Part model, mm, in its own coordinate system. Face numbers are marked on the shaded views. A direction names the side the tool comes from. Round coordinates to 2 decimals unless told otherwise and drop trailing zeros. Write each loop counter-clockwise with the first axis right and the second up, starting at its lowest first coordinate (ties: lowest second). Pieces come first, ordered by that corner, then holes. Notation, with made-up numbers: M 87.25,77.5 L 145.25,77.5 A18 cw 145.25,95.5 Z; hole C 15.25,47 d4. An arc over 180 degrees is marked long. Use a Markdown table: item, result. Add a question column.
1) Slice it at C-C on y = 43.75. Write the cut outline in (x, z), plus the area to 3 significant figures.
2) Two-plate mould, pull along X, no slides. Class the marked faces 4, 5 and 6: released by +X, released by -X, zero draft, split by the parting line, or undercut.
3) Drop flat-ended pins along their axis: P1, Ø4, axis at x = -39.55, y = 45.99, coming from the +Z side; P2, Ø4, axis at x = -41, y = 45.5, coming from the +Z side; P3, Ø2, axis at x = -64.48, y = 45.99, coming from the +Z side; P4, Ø1, axis at x = -54.5, z = 2.5, coming from the +Y side. Give the stop position or say it passes through.
4) Slice it at B-B on x = -48. Write the cut outline in (y, z).
5) Which spindle directions (+Z, -Z, +X, -X, +Y, -Y) get a long thin tool onto all of the face, cutting with end or side? Do the marked faces 1, 2 and 3. Say none if no direction does.
6) Slice it at A-A on y = 45. Write the cut outline in (x, z).
7) Wall check: probe 1 along X at (y, z) = (44.5, 1.45); probe 2 along X at (y, z) = (44, 1.45); probe 3 along Y at (x, z) = (-39, 1.1). Give the ranges that are in metal, low to high.
8) Slice it at D-D on z = 1.5. Write the cut outline in (x, y), plus the area to 3 significant figures.
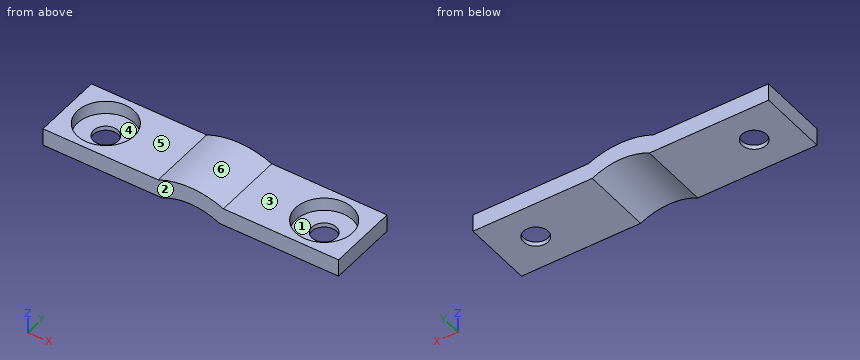
```python
from build123d import *

# Parameters (mm, degrees)
SALIENTE_EXTRUIR3_DEPTH = 4
CROQUIS4_W              = 2
CROQUIS4_H              = 8
SALIENTE_EXTRUIR5_DEPTH = 13.154785
CROQUIS5_R              = 3.25
CORTAR_EXTRUIR1_DEPTH   = 1.5
CORTAR_EXTRUIR2_REACH   = 2.5
CROQUIS6_R              = 1.4


with BuildPart() as part:
    # Croquis3 → Saliente-Extruir3 (new body, symmetric)
    with BuildSketch(Plane(origin=(0, 45.994416346, 0), x_dir=(1, 0, 0), z_dir=(0, 1, 0))):
        with BuildLine():
            ThreePointArc((-58.564503824, 0), (-52.019276555, -2.8), (-45.474049286, 0))
            Line((-45.474049286, 0), (-48.757375269, 0))
            ThreePointArc((-48.757375269, 0), (-52.019276555, -0.8), (-55.281177841, 0))
            Line((-55.281177841, 0), (-58.564503824, 0))
        make_face()
    extrude(amount=SALIENTE_EXTRUIR3_DEPTH, both=True)

    # Croquis4 → Saliente-Extruir5 (add)
    with BuildSketch(Plane(origin=(-68.894276555, 0, 0), x_dir=(0, 0, -1), z_dir=(1, 0, 0))):
        with Locations((-1, 45.994416346)):
            Rectangle(CROQUIS4_W, CROQUIS4_H)
    saliente_extruir5 = extrude(amount=SALIENTE_EXTRUIR5_DEPTH)

    # Simetría1: Saliente-Extruir5 across plane
    add(saliente_extruir5.mirror(Plane(origin=(-52.019276555, 0, 0), x_dir=(0, 0, 1), z_dir=(1, 0, 0))))

    # Croquis5 → Cortar-Extruir1 (cut)
    with BuildSketch(Plane.XY.offset(2)):
        with Locations((-39.554276555, 45.994416346)):
            Circle(CROQUIS5_R)
        with Locations((-64.484276555, 45.994416346)):
            Circle(CROQUIS5_R)
    extrude(amount=-CORTAR_EXTRUIR1_DEPTH, mode=Mode.SUBTRACT)

    # Croquis6 → Cortar-Extruir2 (cut, up to next)
    with BuildSketch(Plane.XY.offset(0.5), mode=Mode.PRIVATE) as cortar_extruir2_sk1:
        with Locations((-39.554276555, 45.994416346)):
            Circle(CROQUIS6_R)
    cortar_extruir2_tool1 = extrude(cortar_extruir2_sk1.sketch, amount=-CORTAR_EXTRUIR2_REACH, mode=Mode.PRIVATE) & part.part
    add(cortar_extruir2_tool1.solids().sort_by_distance((-39.554277, 45.994416, 0.5))[0], mode=Mode.SUBTRACT)
    # Croquis6 → Cortar-Extruir2 (cut, up to next)
    with BuildSketch(Plane.XY.offset(0.5), mode=Mode.PRIVATE) as cortar_extruir2_sk2:
        with Locations((-64.484276555, 45.994416346)):
            Circle(CROQUIS6_R)
    cortar_extruir2_tool2 = extrude(cortar_extruir2_sk2.sketch, amount=-CORTAR_EXTRUIR2_REACH, mode=Mode.PRIVATE) & part.part
    add(cortar_extruir2_tool2.solids().sort_by_distance((-64.484277, 45.994416, 0.5))[0], mode=Mode.SUBTRACT)


solid = part.part
```
Entries:
| question | item | result |
|---|---|---|
| 1 | outline | M -68.89,0 L -55.28,0 A7.05 cw -48.76,0 L -35.14,0 L -35.14,2 L -37.2,2 L -37.2,0.5 L -41.9,0.5 L -41.9,2 L -48.3,2 A9.05 ccw -55.74,2 L -62.13,2 L -62.13,0.5 L -66.83,0.5 L -66.83,2 L -68.89,2 Z |
| 1 | area | 53.9 mm^2 |
| 2 | face 4 | undercut |
| 2 | face 5 | zero draft |
| 2 | face 6 | split by the parting line |
| 3 | P1 | stops at z = 0.5 |
| 3 | P2 | stops at z = 2 |
| 3 | P3 | passes through |
| 3 | P4 | stops at y = 49.99 |
| 4 | outline | M 41.99,0 L 49.99,0 L 49.99,2 L 41.99,2 Z |
| 5 | face 1 | +Z |
| 5 | face 2 | +Z, -Z, +X, -X, -Y |
| 5 | face 3 | +Z, +X, +Y, -Y |
| 6 | outline | M -68.89,0 L -65.47,0 L -65.47,0.5 L -67.58,0.5 L -67.58,2 L -68.89,2 Z; M -63.5,0 L -55.28,0 A7.05 cw -48.76,0 L -40.54,0 L -40.54,0.5 L -42.65,0.5 L -42.65,2 L -48.3,2 A9.05 ccw -55.74,2 L -61.39,2 L -61.39,0.5 L -63.5,0.5 Z; M -38.57,0 L -35.14,0 L -35.14,2 L -36.46,2 L -36.46,0.5 L -38.57,0.5 Z |
| 7 | probe 1 | x = -68.89 to -67.37, -61.6 to -42.44, -36.67 to -35.14 |
| 7 | probe 2 | x = -68.89 to -67.05, -61.92 to -42.12, -36.99 to -35.14 |
| 7 | probe 3 | y = 41.99 to 42.79, 49.2 to 49.99 |
| 8 | outline | M -68.89,41.99 L -35.14,41.99 L -35.14,49.99 L -68.89,49.99 Z; hole C -64.48,45.99 d6.5; hole C -39.55,45.99 d6.5 |
| 8 | area | 204 mm^2 |
